Geometry check sheet. Reference: the model listing, model coordinates, mm. A direction names the side the tool comes from. Give positions to 0.01 mm unless a question says otherwise; leave off trailing zeros. Loops run counter-clockwise (first coordinate to the right, second up) from the corner with the lowest first, then second, coordinate; pieces in that order, holes last. Notation, with made-up numbers: (-17, -11) -> (13, -11) arc R4 cw to (13, -4) -> close; hole circle Ø9 at (-20, -7.75). An arc over 180 degrees is marked (long way). Answer as a JSON object with one key per item and string values.
from build123d import *

# Parameters (mm, degrees)
SKETCH1_W           = 35
SKETCH1_H           = 47.11
BOSS_EXTRUDE1_DEPTH = 4
SKETCH2_R           = 15.25
SKETCH2_R_2         = 11.75
BOSS_EXTRUDE2_DEPTH = 5
BOSS_EXTRUDE3_DEPTH = 60
CUT_EXTRUDE1_START  = -55
CUT_EXTRUDE1_DEPTH  = 55
SKETCH6_R           = 1.7
CUT_EXTRUDE2_DEPTH  = 60
SKETCH7_R           = 8.75
CUT_EXTRUDE3_DEPTH  = 60
FILLET2_R           = 3
FILLET3_R           = 3
SKETCH10_R          = 1.7
CUT_EXTRUDE4_DEPTH  = 71.406590778
FILLET4_R           = 3


with BuildPart() as part:
    # Sketch1 → Boss-Extrude1 (new body)
    with BuildSketch(Plane(origin=(0, 0, 0), x_dir=(1, 0, 0), z_dir=(0, 1, 0))):
        Rectangle(SKETCH1_W, SKETCH1_H)
    extrude(amount=BOSS_EXTRUDE1_DEPTH)

    # Sketch2 → Boss-Extrude2 (add)
    with BuildSketch(Plane.XZ):
        with Locations(Location((0, 0, 0), (0, 0, 90))):
            Circle(SKETCH2_R)
        with Locations(Location((0, 0, 0), (0, 0, 270))):
            Circle(SKETCH2_R_2, mode=Mode.SUBTRACT)
    extrude(amount=BOSS_EXTRUDE2_DEPTH)

    # Sketch3 → Boss-Extrude3 (add)
    with BuildSketch(Plane(origin=(0, 0, 0), x_dir=(-1, 0, 0), z_dir=(0, -1, 0))):
        with BuildLine():
            Line((7.5, 23.555), (7.5, 13.278271725))
            ThreePointArc((7.5, 13.278271725), (5.555361105, 14.202128819), (3.5, 14.842927609))
            Line((3.5, 14.842927609), (3.5, 23.555))
            Line((3.5, 23.555), (7.5, 23.555))
        make_face()
        with BuildLine():
            Line((-7.5, 23.555), (-3.5, 23.555))
            Line((-3.5, 23.555), (-3.5, 14.842927609))
            ThreePointArc((-3.5, 14.842927609), (-5.555361105, 14.202128819), (-7.5, 13.278271725))
            Line((-7.5, 13.278271725), (-7.5, 23.555))
        make_face()
        with BuildLine():
            Line((-7.5, -23.555), (-7.5, -13.278271725))
            ThreePointArc((-7.5, -13.278271725), (-5.555361105, -14.202128819), (-3.5, -14.842927609))
            Line((-3.5, -14.842927609), (-3.5, -23.555))
            Line((-3.5, -23.555), (-7.5, -23.555))
        make_face()
        with BuildLine():
            Line((3.5, -23.555), (3.5, -14.842927609))
            ThreePointArc((3.5, -14.842927609), (5.555361105, -14.202128819), (7.5, -13.278271725))
            Line((7.5, -13.278271725), (7.5, -23.555))
            Line((7.5, -23.555), (3.5, -23.555))
        make_face()
    extrude(amount=BOSS_EXTRUDE3_DEPTH)

    # Sketch5 → Cut-Extrude1 (cut)
    with BuildSketch(Plane.XZ.offset(60).offset(CUT_EXTRUDE1_START)):
        with BuildLine():
            ThreePointArc((-7.5, -13.278271725), (-5.555361105, -14.202128819), (-3.5, -14.842927609))
            Line((-3.5, -14.842927609), (-7.5, -14.842927609))
            Line((-7.5, -14.842927609), (-7.5, -13.278271725))
        make_face()
        with BuildLine():
            Line((7.5, 14.842927609), (3.5, 14.842927609))
            ThreePointArc((3.5, 14.842927609), (5.555361105, 14.202128819), (7.5, 13.278271725))
            Line((7.5, 13.278271725), (7.5, 14.842927609))
        make_face()
        with BuildLine():
            ThreePointArc((3.5, -14.842927609), (5.555361105, -14.202128819), (7.5, -13.278271725))
            Line((7.5, -13.278271725), (7.5, -14.842927609))
            Line((7.5, -14.842927609), (3.5, -14.842927609))
        make_face()
        with BuildLine():
            Line((-3.5, 14.842927609), (-7.5, 14.842927609))
            Line((-7.5, 14.842927609), (-7.5, 13.278271725))
            ThreePointArc((-7.5, 13.278271725), (-5.555361105, 14.202128819), (-3.5, 14.842927609))
        make_face()
    extrude(amount=CUT_EXTRUDE1_DEPTH, mode=Mode.SUBTRACT)

    # Sketch6 → Cut-Extrude2 (cut)
    with BuildSketch(Plane(origin=(7.5, 0, 0), x_dir=(0, 0, -1), z_dir=(1, 0, 0))):
        with Locations((-18.555, -35)):
            Circle(SKETCH6_R)
        with Locations((-18.555, -20)):
            Circle(SKETCH6_R)
        with Locations((-18.555, -50)):
            Circle(SKETCH6_R)
        with Locations((18.555, -50)):
            Circle(SKETCH6_R)
        with Locations((18.555, -35)):
            Circle(SKETCH6_R)
        with Locations((18.555, -20)):
            Circle(SKETCH6_R)
    extrude(amount=-CUT_EXTRUDE2_DEPTH, mode=Mode.SUBTRACT)

    # Sketch7 → Cut-Extrude3 (cut)
    with BuildSketch(Plane(origin=(0, 4, 0), x_dir=(1, 0, 0), z_dir=(0, 1, 0))):
        with Locations(Location((0, 0, 0), (0, 0, 270))):
            Circle(SKETCH7_R)
    extrude(amount=-CUT_EXTRUDE3_DEPTH, mode=Mode.SUBTRACT)

    # Fillet2
    fillet2_edges = [part.edges().sort_by_distance(p)[0] for p in [
        (5.5, -5, -14.842927609),
        (-5.5, -5, -14.842927609),
        (-5.5, -5, 14.842927609),
        (5.5, -5, 14.842927609),
    ]]
    fillet(fillet2_edges, radius=FILLET2_R)

    # Fillet3
    fillet3_edges = [part.edges().sort_by_distance(p)[0] for p in [
        (-5.5, -60, -23.555),
        (5.5, -60, -23.555),
        (5.5, -60, 23.555),
        (-5.5, -60, 23.555),
    ]]
    fillet(fillet3_edges, radius=FILLET3_R)

    # Sketch10 → Cut-Extrude4 (cut, through all)
    with BuildSketch(Plane(origin=(0, 4, 0), x_dir=(1, 0, 0), z_dir=(0, 1, 0))):
        with Locations(Location((-12.5, 18.555, 0), (0, 0, 270))):
            Circle(SKETCH10_R)
        with Locations(Location((12.5, 18.555, 0), (0, 0, 270))):
            Circle(SKETCH10_R)
        with Locations(Location((12.5, -18.555, 0), (0, 0, 270))):
            Circle(SKETCH10_R)
        with Locations(Location((-12.5, -18.555, 0), (0, 0, 270))):
            Circle(SKETCH10_R)
    extrude(amount=-CUT_EXTRUDE4_DEPTH, mode=Mode.SUBTRACT)

    # Fillet4
    fillet4_edges = [part.edges().sort_by_distance(p)[0] for p in [
        (-17.5, 2, -23.555),
        (17.5, 2, -23.555),
        (17.5, 2, 23.555),
        (-17.5, 2, 23.555),
    ]]
    fillet(fillet4_edges, radius=FILLET4_R)


solid = part.part
1) Section check B-B on z = 0. Record the cut outline in (x, y), plus the area to 3 significant figures.
Geometry check:
{"outline": "(-17.5, 0) -> (-15.25, 0) -> (-15.25, -5) -> (-11.75, -5) -> (-11.75, 0) -> (-8.75, 0) -> (-8.75, 4) -> (-17.5, 4) -> close; (8.75, 0) -> (11.75, 0) -> (11.75, -5) -> (15.25, -5) -> (15.25, 0) -> (17.5, 0) -> (17.5, 4) -> (8.75, 4) -> close", "area": "105 mm2"}
2) Section check A-A on y = -50. Count the separate pieces of the cut face and the enclosed holes in it, plus the area to 3 significant figures.
Geometry check:
{"separate pieces": "8", "enclosed holes": "0", "area": "85.0 mm2"}
3) Section check D-D on y = -24. Record the cut outline in (x, z) (3 decimals), plus the area to 3 significant figures.
Geometry check:
{"outline": "(-7.5, -23.555) -> (-3.5, -23.555) -> (-3.5, -14.843) -> (-7.5, -14.843) -> close; (-7.5, 14.843) -> (-3.5, 14.843) -> (-3.5, 23.555) -> (-7.5, 23.555) -> close; (3.5, -23.555) -> (7.5, -23.555) -> (7.5, -14.843) -> (3.5, -14.843) -> close; (3.5, 14.843) -> (7.5, 14.843) -> (7.5, 23.555) -> (3.5, 23.555) -> close", "area": "139 mm2"}
4) Material ranges on line 1 along X through (y, z) = (-44, -19.5); line 2 along X through (y, z) = (1.5, 0); line 3 along Z through (x, y) = (-7, -29.5) (3 decimals), recorded low to high. Write a range as from..to.
Geometry check:
{"line 1": "x = -7.5..-3.5, 3.5..7.5", "line 2": "x = -17.5..-8.75, 8.75..17.5", "line 3": "z = -23.555..-14.843, 14.843..23.555"}
5) Draft check along Z on faces 1 (the face through (5, -60, -18)), 2 (the face through (6, -34, -14.843)), 3 (the face through (-5.472, -18.567, -19.469)), 4 (the face through (16.6, 2, -22.7)). Enter one of: pulls with the +Z half, pulls with the -Z half, needs draft (parallel to the pull), parting line crosses it, or undercut.
Geometry check:
{"face 1": "needs draft", "face 2": "undercut", "face 3": "undercut", "face 4": "pulls with the -Z half"}
6) Tool access check on faces 5 (the face through (-5.918, -5.855, 13.941)), 6 (the face through (-16, 0, 0)), 7 (the face through (0, 0, -19)), 8 (the face through (0, 0, 19)). Record the directions out of +Z, -Z, +X, -X, +Y, -Y that give a thin tool (end or side, any length) a straight path to the whole face; none if there is none.
Geometry check:
{"face 5": "+X, -X, -Y", "face 6": "-X, -Y", "face 7": "-Z, -Y", "face 8": "+Z, -Y"}
7) Section check C-C on x = -5.5. Record the cut outline in (y, z) (3 decimals).
Geometry check:
{"outline": "(-60, -20.555) arc R3 ccw to (-57, -23.555) -> (4, -23.555) -> (4, -6.805) -> (0, -6.805) -> (0, -10.383) -> (-5, -10.383) -> (-5, -11.843) arc R3 cw to (-8, -14.843) -> (-60, -14.843) -> close; (-60, 14.843) -> (-8, 14.843) arc R3 cw to (-5, 11.843) -> (-5, 10.383) -> (0, 10.383) -> (0, 6.805) -> (4, 6.805) -> (4, 23.555) -> (-57, 23.555) arc R3 ccw to (-60, 20.555) -> close; hole circle Ø3.4 at (-50, -18.555); hole circle Ø3.4 at (-50, 18.555); hole circle Ø3.4 at (-35, -18.555); hole circle Ø3.4 at (-35, 18.555); hole circle Ø3.4 at (-20, -18.555); hole circle Ø3.4 at (-20, 18.555)"}
8) Depth check by flat-ended pin: P1, Ø6, axis at x = 14, z = -11, coming from the -Y side; P2, Ø3.5, axis at x = 0.5, z = -19.5, coming from the -Y side; P3, Ø4, axis at y = -35, z = -18.555, coming from the -X side; P4, Ø3, axis at y = -23, z = -12, coming from the +X side. Enter the tip coordinate at first touch or a pass-through.
Geometry check:
{"P1": "stops at y = -5", "P2": "stops at y = 0", "P3": "stops at x = -7.5", "P4": "passes through"}
